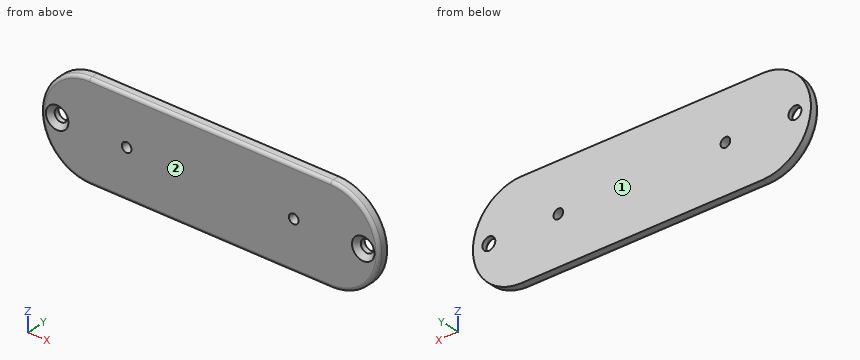
from build123d import *

# Parameters (mm, degrees)
F0_R     = 2
F0_R_2   = 1.5
F1_DEPTH = 3
F2_R     = 1
F3_SIZE  = 1.5
F4_SIZE  = 1.5


with BuildPart() as f1:
    # F0 (on Front) → F1 (new body)
    with BuildSketch(Plane.XZ):
        with BuildLine():
            Line((37.448312, 15.051688), (-37.448312, 15.051688))
            ThreePointArc((-37.448312, 15.051688), (-52.5, 0), (-37.448312, -15.051688))
            Line((-37.448312, -15.051688), (37.448312, -15.051688))
            ThreePointArc((37.448312, -15.051688), (52.5, 0), (37.448312, 15.051688))
        make_face()
        with Locations((-47.538312, 0)):
            Circle(F0_R, mode=Mode.SUBTRACT)
        with Locations((-25.948312, 0)):
            Circle(F0_R_2, mode=Mode.SUBTRACT)
        with Locations((25.948312, 0)):
            Circle(F0_R_2, mode=Mode.SUBTRACT)
        with Locations((47.538312, 0)):
            Circle(F0_R, mode=Mode.SUBTRACT)
    extrude(amount=F1_DEPTH)

    # F2
    f2_edges = [f1.edges().sort_by_distance(p)[0] for p in [
        (0, -3, 15.051688),
        (-52.5, -3, 0),
        (0, -3, -15.051688),
        (52.5, -3, 0),
    ]]
    fillet(f2_edges, radius=F2_R)

    # F3
    f3_edges = [f1.edges().sort_by_distance(p)[0] for p in [
        (-49.538312, -3, 0),
    ]]
    chamfer(f3_edges, length=F3_SIZE)

    # F4
    f4_edges = [f1.edges().sort_by_distance(p)[0] for p in [
        (45.538312, -3, 0),
    ]]
    chamfer(f4_edges, length=F4_SIZE)


solid = f1.part
Could you check a few things on this model? Use its own coordinates, in mm. Face numbers are marked on the shaded views. Round coordinates to 2 decimals unless told otherwise and drop trailing zeros. Order: outer loops, then holes, each group sorted by start corner. A loop starts at its lowest first (then second) coordinate and runs counter-clockwise, first axis right, second up.
Q1. Imagine slicing it at A-A, the plane z = 0. List the corners of the cut face in (x, y) for me.
Geometry says:
outline: (-52.5, -2) arc R1 ccw to (-51.5, -3) - (-51.04, -3) - (-49.54, -1.5) - (-49.54, 0) - (-52.5, 0) - close; (-45.54, -1.5) - (-44.04, -3) - (-27.45, -3) - (-27.45, 0) - (-45.54, 0) - close; (-24.45, -3) - (24.45, -3) - (24.45, 0) - (-24.45, 0) - close; (27.45, -3) - (44.04, -3) - (45.54, -1.5) - (45.54, 0) - (27.45, 0) - close; (49.54, -1.5) - (51.04, -3) - (51.5, -3) arc R1 ccw to (52.5, -2) - (52.5, 0) - (49.54, 0) - close
Q2. Thinking about a two-plate mould opening in Y: for the marked faces 1 and 2, which applies, released by +Y, released by -Y, zero draft, split by the parting line, or undercut?
Geometry says:
face 1: released by +Y
face 2: released by -Y
Q3. Please list where these lines run through material, in increasing order: probe 1 along X at (y, z) = (-1.7, 1); probe 2 along X at (y, z) = (-0.65, 1); probe 3 along Z at (x, y) = (-31, -2.05).
Geometry says:
probe 1: x = -52.47 to -49.5, -45.58 to -27.07, -24.83 to 24.83, 27.07 to 45.58, 49.5 to 52.47
probe 2: x = -52.47 to -49.27, -45.81 to -27.07, -24.83 to 24.83, 27.07 to 45.81, 49.27 to 52.47
probe 3: z = -15.05 to 15.05
Q4. Imagine slicing it at B-B, the plane y = -1. List the corners of the cut face in (x, z) for me, then the cut area to 3 significant figures.
Geometry says:
outline: (-37.45, -15.05) - (37.45, -15.05) arc R15.05 ccw to (37.45, 15.05) - (-37.45, 15.05) arc R15.05 ccw to start; hole circle Ø4 at (-47.54, 0); hole circle Ø3 at (-25.95, 0); hole circle Ø3 at (25.95, 0); hole circle Ø4 at (47.54, 0)
area: 2,930 mm2
